The listing builds one solid part. Answer for the finished solid, in the listing's coordinates (mm). Round coordinates to 2 decimals unless told otherwise and drop trailing zeros. Write each loop counter-clockwise with the first axis right and the second up, starting at its lowest first coordinate (ties: lowest second). Pieces come first, ordered by that corner, then holes. Notation, with made-up numbers: M 66.25,26 L 88.25,26 A18 ccw 88.25,59 Z; hole C 66.25,73.25 d4. An arc over 180 degrees is marked long. Answer as CSV lines item,"result". Start each with the question number.
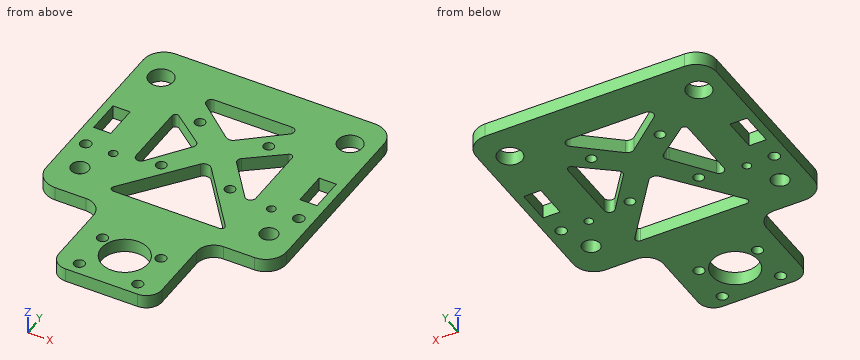
from build123d import *

# Parameters (mm, degrees)
MODEL_R         = 1.25
MODEL_R_2       = 1.6
MODEL_R_3       = 2.55
MODEL_R_4       = 3.556
MODEL_R_5       = 1.5
MODEL_R_6       = 1.55
MODEL_R_7       = 6.75
MODEL_W         = 5
MODEL_H         = 10
EXTRUDE_1_DEPTH = 4


with BuildPart() as part:
    # Model → Бобышка-Вытянуть1 (new body)
    with BuildSketch(Plane.XY):
        with BuildLine():
            Line((-29, 37.192766725), (29, 37.192766725))
            ThreePointArc((29, 37.192766725), (33.242640687, 35.435407412), (35, 31.192766725))
            Line((35, 31.192766725), (35, -19.187803059))
            ThreePointArc((35, -19.187803059), (33.242640687, -23.430443746), (29, -25.187803059))
            Line((29, -25.187803059), (20, -25.187803059))
            ThreePointArc((20, -25.187803059), (16.464466094, -26.652269153), (15, -30.187803059))
            Line((15, -30.187803059), (15, -48.187803059))
            ThreePointArc((15, -48.187803059), (13.681980515, -51.369783574), (10.5, -52.687803059))
            Line((10.5, -52.687803059), (-10.5, -52.687803059))
            ThreePointArc((-10.5, -52.687803059), (-13.681980515, -51.369783574), (-15, -48.187803059))
            Line((-15, -48.187803059), (-15, -30.187803059))
            ThreePointArc((-15, -30.187803059), (-16.464466094, -26.652269153), (-20, -25.187803059))
            Line((-20, -25.187803059), (-29, -25.187803059))
            ThreePointArc((-29, -25.187803059), (-33.242640687, -23.430443746), (-35, -19.187803059))
            Line((-35, -19.187803059), (-35, 31.192766725))
            ThreePointArc((-35, 31.192766725), (-33.242640687, 35.435407412), (-29, 37.192766725))
        make_face()
        with Locations((-22.95502674, -5.842660613)):
            Circle(MODEL_R, mode=Mode.SUBTRACT)
        with Locations((23.04497326, -5.842660613)):
            Circle(MODEL_R, mode=Mode.SUBTRACT)
        with Locations((-30.95502674, -5.842660613)):
            Circle(MODEL_R_2, mode=Mode.SUBTRACT)
        with Locations((31.04497326, -5.842660613)):
            Circle(MODEL_R_2, mode=Mode.SUBTRACT)
        with Locations((-27.5, -15.003318167)):
            Circle(MODEL_R_3, mode=Mode.SUBTRACT)
        with Locations((27.5, 27.008281833)):
            Circle(MODEL_R_4, mode=Mode.SUBTRACT)
        with Locations((-27.5, 27.008281833)):
            Circle(MODEL_R_4, mode=Mode.SUBTRACT)
        with Locations((27.5, -15.003318167)):
            Circle(MODEL_R_3, mode=Mode.SUBTRACT)
        with Locations((-10, -3.997518167)):
            Circle(MODEL_R_5, mode=Mode.SUBTRACT)
        with Locations((10, -3.997518167)):
            Circle(MODEL_R_5, mode=Mode.SUBTRACT)
        with Locations((-10, 16.002481833)):
            Circle(MODEL_R_5, mode=Mode.SUBTRACT)
        with Locations((10, 16.002481833)):
            Circle(MODEL_R_5, mode=Mode.SUBTRACT)
        with Locations((-8.5, -37.087803059)):
            Circle(MODEL_R_6, mode=Mode.SUBTRACT)
        with Locations((8.5, -37.087803059)):
            Circle(MODEL_R_6, mode=Mode.SUBTRACT)
        with Locations((-8.5, -49.087803059)):
            Circle(MODEL_R_6, mode=Mode.SUBTRACT)
        with Locations((0, -40.687803059)):
            Circle(MODEL_R_7, mode=Mode.SUBTRACT)
        with Locations((8.5, -49.087803059)):
            Circle(MODEL_R_6, mode=Mode.SUBTRACT)
        with Locations((-30, 6.002481833)):
            Rectangle(MODEL_W, MODEL_H, mode=Mode.SUBTRACT)
        with Locations((30, 6.002481833)):
            Rectangle(MODEL_W, MODEL_H, mode=Mode.SUBTRACT)
        with BuildLine():
            Line((-15.452005485, -19.187803059), (15.452005485, -19.187803059))
            ThreePointArc((15.452005485, -19.187803059), (16.350604725, -18.626573394), (16.240562864, -17.572841873))
            Line((16.240562864, -17.572841873), (1.577114757, 1.229922372))
            ThreePointArc((1.577114757, 1.229922372), (0, 2), (-1.577114757, 1.229922372))
            Line((-1.577114757, 1.229922372), (-16.240562864, -17.572841873))
            ThreePointArc((-16.240562864, -17.572841873), (-16.350604725, -18.626573394), (-15.452005485, -19.187803059))
        make_face(mode=Mode.SUBTRACT)
        with BuildLine():
            Line((6.179376111, 6.169053374), (14.817163932, -4.907078707))
            ThreePointArc((14.817163932, -4.907078707), (16.487722205, -5.403131571), (17.5, -3.984636928))
            Line((17.5, -3.984636928), (17.5, 14.851722882))
            ThreePointArc((17.5, 14.851722882), (16.938770335, 15.750322122), (15.885038814, 15.640280261))
            Line((15.885038814, 15.640280261), (6.4397704, 8.274331221))
            ThreePointArc((6.4397704, 8.274331221), (5.873555937, 7.275621721), (6.179376111, 6.169053374))
        make_face(mode=Mode.SUBTRACT)
        with BuildLine():
            Line((-17.5, 14.851722882), (-17.5, -3.768193645))
            ThreePointArc((-17.5, -3.768193645), (-16.466952403, -5.193660394), (-14.790726063, -4.655693811))
            Line((-14.790726063, -4.655693811), (-6.96856736, 6.002481833))
            Line((-6.96856736, 6.002481833), (-6.589337275, 6.488764039))
            ThreePointArc((-6.589337275, 6.488764039), (-6.283517101, 7.595332385), (-6.849731564, 8.594041886))
            Line((-6.849731564, 8.594041886), (-15.885038814, 15.640280261))
            ThreePointArc((-15.885038814, 15.640280261), (-16.938770335, 15.750322122), (-17.5, 14.851722882))
        make_face(mode=Mode.SUBTRACT)
        with BuildLine():
            Line((11.296355011, 25.692278611), (-11.296355011, 25.692278611))
            ThreePointArc((-11.296355011, 25.692278611), (-12.707256514, 24.701549606), (-12.254396629, 23.038087873))
            Line((-12.254396629, 23.038087873), (-1.277388824, 13.926569315))
            ThreePointArc((-1.277388824, 13.926569315), (0, 13.465490298), (1.277388824, 13.926569315))
            Line((1.277388824, 13.926569315), (12.254396629, 23.038087873))
            ThreePointArc((12.254396629, 23.038087873), (12.707256514, 24.701549606), (11.296355011, 25.692278611))
        make_face(mode=Mode.SUBTRACT)
    extrude(amount=EXTRUDE_1_DEPTH)


solid = part.part
Q1. Find section A-A (x = 0). Determine the outline of the cut face in (y, z).
Q2. Each of these flat-tipped pins is pushed along its axis until it touches: P1, Ø1, axis at x = 13, y = -1.5, coming from the +Z side; P2, Ø1, axis at y = -32.5, z = 0.5, coming from the -X side. Where does it stop, or does it pass through?
Q3. Straight lines are drawn through the part: L1, parallel to X at y = 12, z = 2.3; L2, parallel to Y at x = -1.5, z = 0.7; L3, parallel to Y at x = 27, z = 0.2. For each, find the intervals that lie inside material, in ascending order.
Q4. Find section B-B (z = 2.7). Count the separate pieces of the cut face and the enclosed holes in it, plus the area to 3 significant figures.
Reported:
1,outline,"M -52.69,0 L -47.44,0 L -47.44,4 L -52.69,4 Z; M -33.94,0 L -19.19,0 L -19.19,4 L -33.94,4 Z; M 2,0 L 13.47,0 L 13.47,4 L 2,4 Z; M 25.69,0 L 37.19,0 L 37.19,4 L 25.69,4 Z"
2,P1,"passes through"
2,P2,"stops at x = -15"
3,L1,"x = -35 to -17.5, -11.22 to 11.22, 17.5 to 35"
3,L2,"y = -52.69 to -47.27, -34.11 to -19.19, 1.32 to 14.11, 25.69 to 37.19"
3,L3,"y = -25.19 to -17.5, -12.5 to 23.49, 30.53 to 37.19"
4,separate pieces,"1"
4,enclosed holes,"23"
4,area,"3,840 mm2"
